Verification items for this drawing (mm, ordinates from the low corner). Give positions to 0.01 mm unless a question says otherwise; leave off trailing zeros. Order: outer loops, then holes, each group sorted by start corner. A loop starts at its lowest first (then second) coordinate and runs counter-clockwise, first axis right, second up. Notation, with made-up numbers: M -13,78.25 L -5,78.25 A6 ccw -5,87.25 Z; hole C -14.5,73 d6. An arc over 180 degrees is marked long. Return JSON: item names as keys, results as strings. Group by question number.
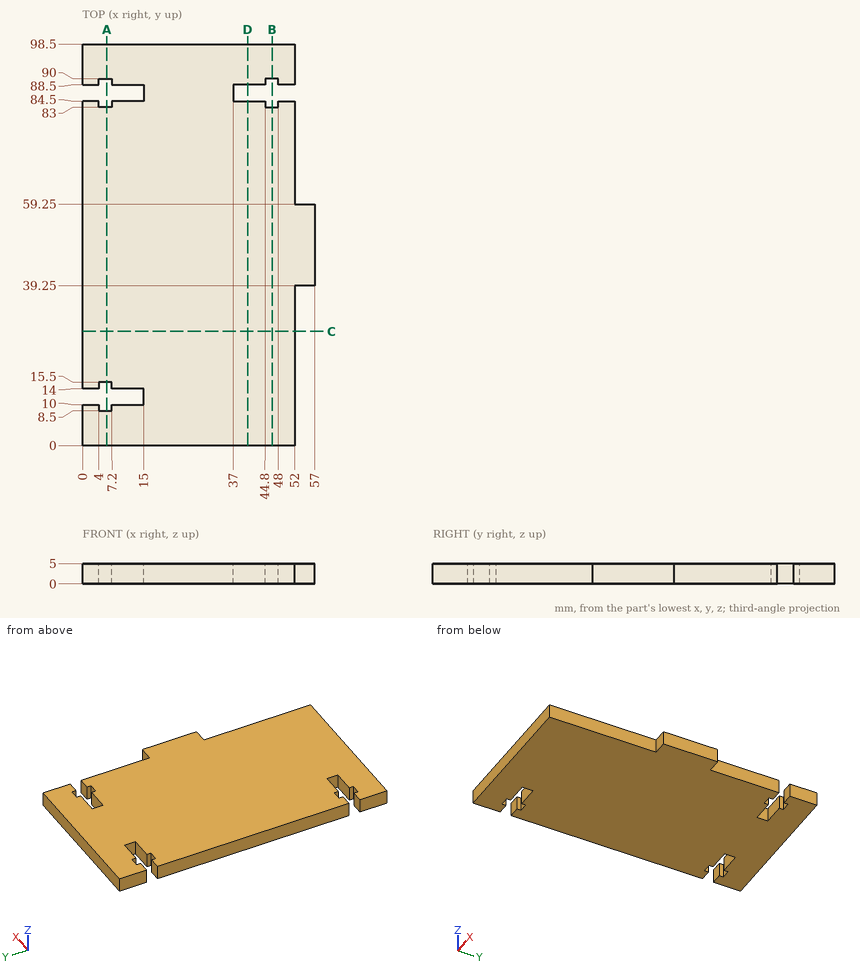
1) Sectioned sample at B-B on x = 46.5. Record the boundary of the cut face in (y, z).
2) Sectioned sample at A-A on x = 6. Record the boundary of the cut face in (y, z).
3) Sectioned sample at C-C on y = 28. Record the boundary of the cut face in (x, z).
4) Depth check by flat-ended pin: P1, Ø1.2, axis at y = 11.5, z = 3.5, coming from the -X side; P2, Ø2.5, axis at x = 55, z = 3.5, coming from the +Y side; P3, Ø1.5, axis at y = 16.5, z = 4, coming from the +X side. Enter the tip coordinate at first touch or a pass-through.
5) Material ranges on line 1 along Y through (x, z) = (13.5, 1.1); line 2 along Y through (x, z) = (40.5, 4.4); line 3 along X through (y, z) = (73, 1.3), recorded low to high.
6) Sectioned sample at D-D on x = 40.5. Record the boundary of the cut face in (y, z), then the cut area to 4 significant figures.
Reply:
{
 "1": {"outline": "M 0,0 L 83,0 L 83,5 L 0,5 Z; M 90,0 L 98.5,0 L 98.5,5 L 90,5 Z"},
 "2": {"outline": "M 0,0 L 8.5,0 L 8.5,5 L 0,5 Z; M 15.5,0 L 83,0 L 83,5 L 15.5,5 Z; M 90,0 L 98.5,0 L 98.5,5 L 90,5 Z"},
 "3": {"outline": "M 0,0 L 52,0 L 52,5 L 0,5 Z"},
 "4": {"P1": "x = 15", "P2": "y = 59.25", "P3": "x = 52"},
 "5": {"line 1": "0 to 10, 14 to 84.5, 88.5 to 98.5", "line 2": "0 to 84.5, 88.5 to 98.5", "line 3": "0 to 52"},
 "6": {"outline": "M 0,0 L 84.5,0 L 84.5,5 L 0,5 Z; M 88.5,0 L 98.5,0 L 98.5,5 L 88.5,5 Z", "area": "472.5 mm^2"}
}
